The listing builds one solid part. Answer for the finished solid, in the listing's coordinates (mm). A direction names the side the tool comes from. Round coordinates to 2 decimals unless told otherwise and drop trailing zeros. Write each loop counter-clockwise with the first axis right and the second up, starting at its lowest first coordinate (ties: lowest second). Pieces come first, ordered by that corner, then holes.
Item 1: For a pull along Z with two mould halves and no side action, classify faces 5 (the face through (-1, -3.25, 10)), 6 (the face through (0, 0, 19.3)), 7 (the face through (-1, -23.05, 10)) as +Z half, -Z half, draft (parallel to the pull), parting line (faces both ways), or undercut.
Item 2: Find section B-B on x = 0.25. Give the vertices of the cut face in (y, z).
Item 3: Find section A-A on z = 12.5. Give the vertices of the cut face in (x, y), then the cut area to 3 significant figures.
Item 4: A tool of negligible diameter and unlimited length cuts with its end or side. For faces 1 (the face through (0, 7, 2)), 2 (the face through (1.8, -17, 10)), 3 (the face through (-5.8, -7, 10)), 4 (the face through (-4.2, -17, 10)), from which of +Z, -Z, +X, -X, +Y, -Y can it reach the whole face along a straight path? Write none if from no direction.
Item 5: Find section D-D on x = 4.25. Give the vertices of the cut face in (y, z), then the cut area to 3 significant figures.
Item 6: Each of these flat-tipped pins is pushed along its axis until it touches: pin 1 (10 mm diameter, centred on y = -17, z = 12, fed in from -X); pin 2 (1.5 mm diameter, centred on x = -4.5, z = 14, fed in from -Y); pin 3 (6.5 mm diameter, centred on y = -18.5, z = 9, fed in from +X). Where does it stop, or does it pass through?
Item 7: Find section C-C on y = 0.5. Give the vertices of the cut face in (x, z), then the cut area to 3 significant figures.
Item 8: Find the intervals of material crossed by probe 1 along Z at (x, y) = (-2, 4.5); probe 2 along X at (y, z) = (17, 8.5); probe 3 along Y at (x, z) = (-1, 16.5), in increasing order.
```python
from build123d import *

# Parameters (mm, degrees)
SALIENTE_EXTRUIR1_DEPTH = 19.3
CROQUIS2_W              = 15.3
CROQUIS2_H              = 26.3
CORTAR_EXTRUIR1_DEPTH   = 9.3


with BuildPart() as part:
    # Croquis1 → Saliente-Extruir1 (new body)
    with BuildSketch(Plane.XY):
        with BuildLine():
            Line((5.8, 23.05), (2.4, 23.05))
            Line((2.4, 23.05), (-5.8, -0.85))
            Line((-5.8, -0.85), (-5.8, -10.609737321))
            ThreePointArc((-5.8, -10.609737321), (-5.505459406, -11.318487649), (-4.795345946, -11.609726491))
            Line((-4.795345946, -11.609726491), (-4.702327027, -11.609293571))
            ThreePointArc((-4.702327027, -11.609293571), (-4.347270297, -11.754912992), (-4.2, -12.109288156))
            Line((-4.2, -12.109288156), (-4.2, -21.05))
            ThreePointArc((-4.2, -21.05), (-3.614213562, -22.464213562), (-2.2, -23.05))
            Line((-2.2, -23.05), (-0.2, -23.05))
            ThreePointArc((-0.2, -23.05), (1.214213562, -22.464213562), (1.8, -21.05))
            Line((1.8, -21.05), (1.8, -13.106955688))
            ThreePointArc((1.8, -13.106955688), (2.239339828, -12.046295517), (3.3, -11.606955688))
            Line((3.3, -11.606955688), (3.8, -11.606955688))
            ThreePointArc((3.8, -11.606955688), (5.214213562, -11.021169251), (5.8, -9.606955688))
            Line((5.8, -9.606955688), (5.8, 23.05))
        make_face()
    extrude(amount=SALIENTE_EXTRUIR1_DEPTH)

    # Croquis2 → Cortar-Extruir1 (cut)
    with BuildSketch(Plane.ZY.offset(5.8)):
        with Locations((9.65, 9.9)):
            Rectangle(CROQUIS2_W, CROQUIS2_H)
    extrude(amount=-CORTAR_EXTRUIR1_DEPTH, mode=Mode.SUBTRACT)


solid = part.part
```
Check values:
1. face 5: undercut
1. face 6: +Z half
1. face 7: draft
2. outline: (-23, 0) - (16.78, 0) - (16.78, 2) - (-3.25, 2) - (-3.25, 17.3) - (16.78, 17.3) - (16.78, 19.3) - (-23, 19.3) - close
3. outline: (-5.8, -10.61) arc R1 ccw to (-4.8, -11.61) - (-4.7, -11.61) arc R0.5 cw to (-4.2, -12.11) - (-4.2, -21.05) arc R2 ccw to (-2.2, -23.05) - (-0.2, -23.05) arc R2 ccw to (1.8, -21.05) - (1.8, -13.11) arc R1.5 cw to (3.3, -11.61) - (3.8, -11.61) arc R2 ccw to (5.8, -9.61) - (5.8, 23.05) - (3.5, 23.05) - (3.5, -3.25) - (-5.8, -3.25) - close
3. area: 224 mm2
4. face 1: -X, +Y
4. face 2: +Z, -Z, +X, -Y
4. face 3: +Z, -Z, -X, +Y, -Y
4. face 4: +Z, -Z, -X, -Y
5. outline: (-11.56, 0) - (23.05, 0) - (23.05, 19.3) - (-11.56, 19.3) - close
5. area: 668 mm2
6. pin 1: stops at x = -4.21
6. pin 2: stops at y = -22.31
6. pin 3: stops at x = 1.8
7. outline: (-5.34, 0) - (5.8, 0) - (5.8, 19.3) - (-5.34, 19.3) - (-5.34, 17.3) - (3.5, 17.3) - (3.5, 2) - (-5.34, 2) - close
7. area: 79.7 mm2
8. probe 1: z = 0 to 2, 17.3 to 19.3
8. probe 2: x = 3.5 to 5.8
8. probe 3: y = -23.05 to -3.25
